Geometry: final body of the model. Coordinates: model frame, mm. Face numbers are marked on the shaded views. A direction names the side the tool comes from. Round coordinates to 2 decimals unless told otherwise and drop trailing zeros. Write each loop counter-clockwise with the first axis right and the second up, starting at its lowest first coordinate (ties: lowest second). Pieces come first, ordered by that corner, then holes. Notation, with made-up numbers: (23, -32) -> (35, -32) arc R22 ccw to (35, 2) -> close; hole circle Ø2 at (46.5, -23). An arc over 180 degrees is marked (long way). One line per item, written item: value. Start each with the question number.
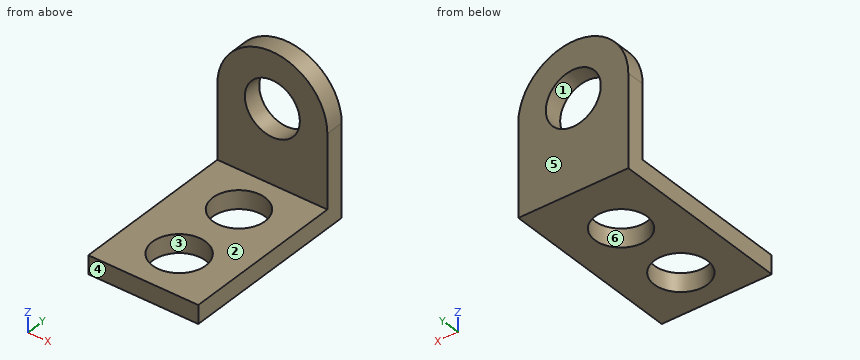
from build123d import *

# Parameters (mm, degrees)
F0_R     = 150
F1_DEPTH = 100
F0_W     = 600
F0_H     = 100
F2_DEPTH = 1000
F3_R     = 142.755464
F3_R_2   = 144.928128
F4_DEPTH = 100


with BuildPart() as f1:
    # F0 (on Front) → F1 (new body)
    with BuildSketch(Plane.XZ):
        with BuildLine():
            Line((300, -400), (300, 0))
            ThreePointArc((300, 0), (0, 300), (-300, 0))
            Line((-300, 0), (-300, -400))
            Line((-300, -400), (300, -400))
        make_face()
        Circle(F0_R, mode=Mode.SUBTRACT)
    extrude(amount=F1_DEPTH)

    # F0 (on Front) → F2 (join)
    with BuildSketch(Plane.XZ):
        with Locations((0, -450)):
            Rectangle(F0_W, F0_H)
    extrude(amount=F2_DEPTH)

    # F3 (on face) → F4 (cut)
    with BuildSketch(Plane.XY.offset(-400)):
        with Locations((0, -333)):
            Circle(F3_R)
        with Locations((0, -750)):
            Circle(F3_R_2)
    extrude(amount=-F4_DEPTH, mode=Mode.SUBTRACT)


solid = f1.part
(1) Section query B-B (x = 0). Output: boundary loops of the cut face in (y, z), and give its area (3 significant figures).
(2) Pull-direction query (Y, two-part tool) for the marked faces 3, 4, 5 and 6; classes: pulls with the +Y half, pulls with the -Y half, needs draft (parallel to the pull), parting line crosses it, or undercut.
(3) Line query: probe 1 along Y at (x, z) = (0, -449); probe 2 along Z at (x, y) = (0, -46); probe 3 along X at (y, z) = (-84, -126). Output: solid intervals per line, ascending.
(4) Section query D-D (x = 74.5). Output: boundary loops of the cut face in (y, z).
(5) Section query A-A (y = -750). Output: boundary loops of the cut face in (x, z), and give its area (3 significant figures).
(6) Pin query (flat end, axial travel): pin 1 (1 mm diameter, centred on x = -203, y = -837, fed in from +Z). Return the tip coordinate at first contact, or that it passes through.
(7) Section query C-C (z = -61). Output: boundary loops of the cut face in (x, y), and give its area (3 significant figures).
(8) Set-up query: the marked faces 1 and 2. Return all of +Z, -Z, +X, -X, +Y, -Y with unobstructed straight access to the full face (end or side cutting, diameter ignored); none if empty.
Results list:
1. outline: (-1000, -500) -> (-894.93, -500) -> (-894.93, -400) -> (-1000, -400) -> close; (-605.07, -500) -> (-475.76, -500) -> (-475.76, -400) -> (-605.07, -400) -> close; (-190.24, -500) -> (0, -500) -> (0, -150) -> (-100, -150) -> (-100, -400) -> (-190.24, -400) -> close; (-100, 150) -> (0, 150) -> (0, 300) -> (-100, 300) -> close
1. area: 82,500 mm^2
2. face 3: undercut
2. face 4: pulls with the -Y half
2. face 5: pulls with the +Y half
2. face 6: undercut
3. probe 1: y = -1000 to -894.93, -605.07 to -475.76, -190.24 to 0
3. probe 2: z = -500 to -150, 150 to 300
3. probe 3: x = -300 to -81.39, 81.39 to 300
4. outline: (-1000, -500) -> (-874.31, -500) -> (-874.31, -400) -> (-1000, -400) -> close; (-625.69, -500) -> (-454.77, -500) -> (-454.77, -400) -> (-625.69, -400) -> close; (-211.23, -500) -> (0, -500) -> (0, -130.19) -> (-100, -130.19) -> (-100, -400) -> (-211.23, -400) -> close; (-100, 130.19) -> (0, 130.19) -> (0, 290.6) -> (-100, 290.6) -> close
5. outline: (-300, -500) -> (-144.93, -500) -> (-144.93, -400) -> (-300, -400) -> close; (144.93, -500) -> (300, -500) -> (300, -400) -> (144.93, -400) -> close
5. area: 31,000 mm^2
6. pin 1: stops at z = -400
7. outline: (-300, -100) -> (-137.04, -100) -> (-137.04, 0) -> (-300, 0) -> close; (137.04, -100) -> (300, -100) -> (300, 0) -> (137.04, 0) -> close
7. area: 32,600 mm^2
8. face 1: +Y, -Y
8. face 2: +Z, +X, -X, -Y
